Source: CAD feature listing. Evaluate the final solid. Frame: model axes, mm. Face numbers are marked on the shaded views. A direction names the side the tool comes from. Round coordinates to 2 decimals unless told otherwise and drop trailing zeros. Write each loop counter-clockwise with the first axis right and the second up, starting at its lowest first coordinate (ties: lowest second). Pieces come first, ordered by that corner, then holes. Notation, with made-up numbers: M 4.5,-34 L 21.5,-34 A14 ccw 21.5,-16 Z; hole C -5.5,31 d4. An arc over 180 degrees is marked long. Answer in a Markdown table with one row per item. Add a question column.
Item 1: Cut plane A-A on z = 0. Give the number of separate pieces and of enclosed holes in the cut face, and give its area (3 significant figures).
Item 2: Material intervals for probe 1 along Y at (x, z) = (128.25, 0); probe 2 along Z at (x, y) = (-251.5, 0); probe 3 along Y at (x, z) = (-128.5, -9), sorted ascending.
Item 3: Contact query for flat-ended pins moving along their axis: pin 1 (2 mm diameter, centred on x = -68.5, z = 1, fed in from -Y); pin 2 (20 mm diameter, centred on y = -40, z = 69.28, fed in from -X); pin 3 (2 mm diameter, centred on x = -190, z = -34, fed in from -Y). Output: stop coordinate, or through.
Item 4: Cut plane B-B on x = -221.5. Return loops of the section in (y, z).
Item 5: Mould query, pull axis Y, two halves, no side actions, for the marked faces 1, 2 and 3. Classes: released by +Y, released by -Y, zero draft, split by the parting line, or undercut.
Item 6: Cut plane D-D on x = -28.5. Return loops of the section in (y, z).
Item 7: Set-up query: the marked faces 4 and 5. Return all of +Z, -Z, +X, -X, +Y, -Y with unobstructed straight access to the full face (end or side cutting, diameter ignored); none if empty.
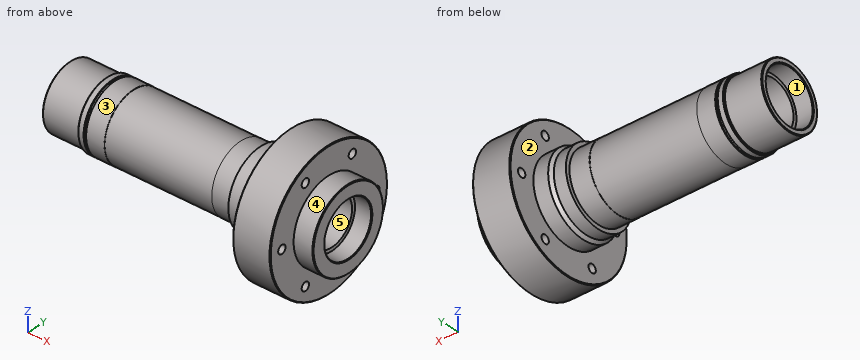
from build123d import *

# Parameters (mm, degrees)
SMUSSO1_SIZE                = 1
SMUSSO2_SIZE                = 1
SCHIZZO6_R                  = 6.25
TAGLIO_ESTRUSIONE1_DEPTH    = 56
RIPETIZIONECIRCOLARE1_COUNT = 6


with BuildPart() as part:
    # Schizzo1 → Rivoluzione1 (revolve)
    with BuildSketch(Plane.XY):
        Polygon((13.630317818, 50), (-16.369682182, 50), (-16.369682182, 49.75), (-176.369682182, 49.75), (-176.369682182, 50), (-203.869682182, 50), (-203.869682182, 48.25), (-207.619682182, 48.25), (-207.619682182, 50), (-216.369682182, 50), (-216.369682182, 47.5), (-271.369682182, 47.5), (-271.369682182, 40), (-246.369682182, 40), (-246.369682182, 35), (118.630317818, 35), (118.630317818, 40), (143.630317818, 40), (143.630317818, 60), (114.630317818, 60), (114.630317818, 100), (58.630317818, 100), (58.630317818, 60), (36.630317818, 60), (31.672388014, 56), (13.630317818, 56), align=None)
    revolve(axis=Axis((0, 0, 0), (-1, 0, 0)))

    # Smusso1
    smusso1_edges = [part.edges().sort_by_distance(p)[0] for p in [
        (58.630317818, -100, 0),
        (114.630317818, -100, 0),
        (143.630317818, -60, 0),
    ]]
    chamfer(smusso1_edges, length=SMUSSO1_SIZE)

    # Smusso2
    smusso2_edges = [part.edges().sort_by_distance(p)[0] for p in [
        (143.630317818, -40, 0),
        (-271.369682182, -40, 0),
        (-271.369682182, -47.5, 0),
        (-216.369682182, -50, 0),
    ]]
    chamfer(smusso2_edges, length=SMUSSO2_SIZE)

    # Schizzo6 → Taglio-Estrusione1 (cut)
    with BuildSketch(Plane(origin=(114.630317818, 0, 0), x_dir=(0, 0, -1), z_dir=(1, 0, 0))):
        with Locations(Location((0, -80, 0), (0, 0, 90))):
            Circle(SCHIZZO6_R)
    taglio_estrusione1 = extrude(amount=-TAGLIO_ESTRUSIONE1_DEPTH, mode=Mode.SUBTRACT)

    # RipetizioneCircolare1: Taglio-Estrusione1 ×6 about axis
    ripetizionecircolare1_axis = Axis((0, 0, 0), (1, 0, 0))
    for i in range(1, RIPETIZIONECIRCOLARE1_COUNT):
        add(taglio_estrusione1.rotate(ripetizionecircolare1_axis, i * 360 / RIPETIZIONECIRCOLARE1_COUNT), mode=Mode.SUBTRACT)


solid = part.part
Results below:
| question | item | result |
|---|---|---|
| 1 | separate pieces | 4 |
| 1 | enclosed holes | 0 |
| 1 | area | 17,100 mm2 |
| 2 | probe 1 | -60 to -40, 40 to 60 |
| 2 | probe 2 | -47.5 to -40, 40 to 47.5 |
| 2 | probe 3 | -48.93 to -33.82, 33.82 to 48.93 |
| 3 | pin 1 | y = -49.75 |
| 3 | pin 2 | x = 58.63 |
| 3 | pin 3 | y = -37.56 |
| 4 | outline | C 0,0 d95; hole C 0,0 d70 |
| 5 | face 1 | undercut |
| 5 | face 2 | zero draft |
| 5 | face 3 | split by the parting line |
| 6 | outline | C 0,0 d99.5; hole C 0,0 d70 |
| 7 | face 4 | +X |
| 7 | face 5 | +X, -X |
